```python
from build123d import *

# Parameters (mm, degrees)
SKETCH1_LINK1_R     = 20
BOSS_EXTRUDE1_DEPTH = 40
SKETCH2_LINK1_R     = 20
CUT_EXTRUDE1_DEPTH  = 40


with BuildPart() as part:
    # sketch1_link1 → Boss-Extrude1 (new body, symmetric)
    with BuildSketch(Plane.XY):
        with BuildLine():
            Line((-40, 0), (-40, 121.875))
            ThreePointArc((-40, 121.875), (0, 161.875), (40, 121.875))
            Line((40, 121.875), (40, 0))
            Line((40, 0), (0, 0))
            Line((0, 0), (-40, 0))
        make_face()
        with Locations((0, 121.875)):
            Circle(SKETCH1_LINK1_R, mode=Mode.SUBTRACT)
    extrude(amount=BOSS_EXTRUDE1_DEPTH, both=True)

    # sketch2_link1 → Cut-Extrude1 (cut)
    with BuildSketch(Plane(origin=(0, 0, 0), x_dir=(1, 0, 0), z_dir=(0, 1, 0))):
        Circle(SKETCH2_LINK1_R)
    extrude(amount=CUT_EXTRUDE1_DEPTH, mode=Mode.SUBTRACT)


solid = part.part
```
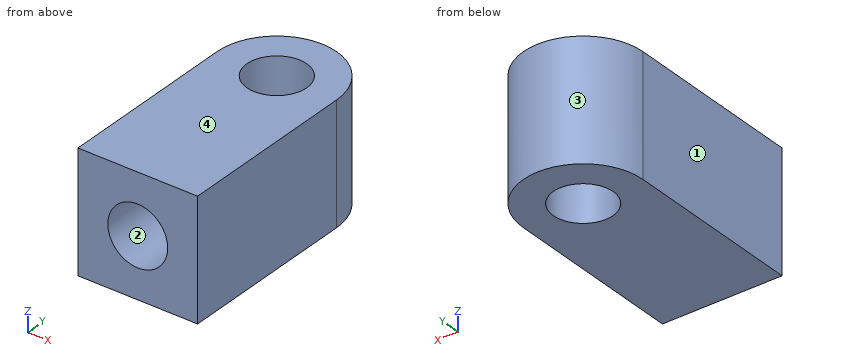
CAD build for the part. Positions are in the model's coordinates, mm. Face numbers are marked on the shaded views. Round coordinates to 2 decimals unless told otherwise and drop trailing zeros. Order: outer loops, then holes, each group sorted by start corner. A loop starts at its lowest first (then second) coordinate and runs counter-clockwise, first axis right, second up. Notation, with made-up numbers: (67.25, 37.5) -> (86.25, 37.5) arc R21 cw to (86.25, 41.5) -> close; hole circle Ø1 at (31.5, 72.5). An arc over 180 degrees is marked (long way). Write item = value, one per line.
(1) Pull direction X, two halves, no side cores. Call the marked faces 1, 2, 3 and 4: +X half, -X half, draft (parallel to the pull), parting line (faces both ways), or undercut.
Answers follow:
face_1 = -X half
face_2 = undercut
face_3 = parting line
face_4 = draft
(2) Cut at B-B (x = 0). Write the cut outline in (y, z) (3 decimals), plus the area to 3 significant figures.
Answers follow:
outline = (0, -40) -> (101.875, -40) -> (101.875, 40) -> (0, 40) -> (0, 20) -> (40, 20) -> (40, -20) -> (0, -20) -> close; (141.875, -40) -> (161.875, -40) -> (161.875, 40) -> (141.875, 40) -> close
area = 8,150 mm²
(3) Cut at C-C (y = 130.5). Write the cut outline in (x, z).
Answers follow:
outline = (-39.06, -40) -> (-18.04, -40) -> (-18.04, 40) -> (-39.06, 40) -> close; (18.04, -40) -> (39.06, -40) -> (39.06, 40) -> (18.04, 40) -> close
(4) Cut at A-A (z = 0). Write the cut outline in (x, y) (3 decimals), plus the area to 3 significant figures.
Answers follow:
outline = (-40, 0) -> (-20, 0) -> (-20, 40) -> (20, 40) -> (20, 0) -> (40, 0) -> (40, 121.875) arc R40 ccw to (-40, 121.875) -> close; hole circle Ø40 at (0, 121.875)
area = 9,410 mm²
(5) Flat gauge pins, fed straight in: P1, Ø12, axis at y = 129, z = -29, coming from the -X side; P2, Ø8, axis at x = 19.5, z = 14.5, coming from the +Y side. Where does each tip first touch, or does it go through?
Answers follow:
P1 = -39.98
P2 = 158.75
(6) Drill centre lines: L1, parallel to Z at x = 0, y = 9; L2, parallel to Y at x = 0, z = -6 (3 decimals). Where is each one in solid material? Low to high.
Answers follow:
L1 = -40 to -20, 20 to 40
L2 = 40 to 101.875, 141.875 to 161.875
(7) Cut at D-D (y = 25). Write the cut outline in (x, z), plus the area to 3 significant figures.
Answers follow:
outline = (-40, -40) -> (40, -40) -> (40, 40) -> (-40, 40) -> close; hole circle Ø40 at (0, 0)
area = 5,140 mm²
